Autodesk Inventor part; units mm, degrees
ref_plane "YZ Plane" through (0, 0, 0) normal (1, 0, 0) x (0, 1, 0)
ref_plane "XZ Plane" through (0, 0, 0) normal (0, 1, 0) x (-1, 0, 0)
ref_plane "XY Plane" through (0, 0, 0) normal (0, 0, 1) x (1, 0, 0)
sketch "Sketch1" plane through (0, 0, 0) normal (0, 1, 0) x (-1, 0, 0)
  line L0 (0, 0) -> (85.48, 0)
  line L1 (85.48, 0) -> (85.48, -127.76)
  line L2 (85.48, -127.76) -> (0, -127.76)
  line L3 (0, -127.76) -> (0, 0)
  line L4 (0, 0) -> (7.0711, -7.0711)
  line L5 (0, 0) -> (10, 0) construction
  circle A0 centre (7.0711, -7.0711) radius 4.7625
  dimension "d0" = 85.48
  dimension "d1" = 127.76
  dimension "offsetDiag" = 10
  dimension "d3" = 45
  dimension "d4" = 9.525
extrude "Extrusion1" add sketch "Sketch1" along normal blind 6.35 contours L0 L1 L2 L3 | A0
sketch "Sketch3" plane through (0, 6.35, 0) normal (0, 1, 0) x (1, 0, 0)
  line L0 (0, 0) -> (0, 127.76)
  line L1 (0, 0) -> (-2.3876, 0)
  line L2 (-2.3876, 0) -> (-2.3876, 9.8298)
  line L3 (-2.3876, 9.8298) -> (0, 9.8298)
  line L4 (0, 9.8298) -> (0, 0)
  line L5 (-2.3876, 9.8298) -> (-28.2876, 9.8298)
  line L6 (-28.2876, 9.8298) -> (-28.2876, 35.7298)
  line L7 (-28.2876, 35.7298) -> (-2.3876, 35.7298)
  line L8 (-2.3876, 35.7298) -> (-2.3876, 9.8298)
  line L9 (-28.2876, 35.7298) -> (-29.2876, 35.7298)
  line L10 (-29.2876, 35.7298) -> (-29.2876, 36.7298)
  line L11 (-29.2876, 36.7298) -> (-28.2876, 36.7298)
  line L12 (-28.2876, 36.7298) -> (-28.2876, 35.7298)
  dimension "d23" = 2.3876
  dimension "d24" = 9.8298
  dimension "d25" = 25.9
  dimension "d26" = 25.9
  dimension "d27" = 1
  dimension "d28" = 1
extrude "Extrusion2" cut sketch "Sketch3" against normal blind 1 contours L5 L6 L7 L8
pattern_linear "Rectangular Pattern2" count 3 spacing 27.4 along (-1, 0, 0) count 4 spacing 27.4 along (0, 0, -1) of "Extrusion2"
properties part number "inch substrate rack"
The listing builds one solid part. Answer for the finished solid, in the listing's coordinates (mm). A direction names the side the tool comes from. Give positions to 0.01 mm unless a question says otherwise; leave off trailing zeros. Order: outer loops, then holes, each group sorted by start corner. A loop starts at its lowest first (then second) coordinate and runs counter-clockwise, first axis right, second up.
Item 1: Find the intervals of material crossed by probe 1 along Z at (x, y) = (-26.5, 6); probe 2 along Y at (x, z) = (-10.5, -114), in increasing order.
From the geometry:
probe 1: z = -127.76 to -117.93, -92.03 to -90.53, -64.63 to -63.13, -37.23 to -35.73, -9.83 to 0
probe 2: y = 0 to 5.35
Item 2: Which of the six approach directions +Z, -Z, +X, -X, +Y, -Y give full straight-line access (tool end or side, diameter ignored) to faces 1 (the face through (-43, 5.35, -78)), 2 (the face through (-43, 3, -127.76))?
From the geometry:
face 1: +Y
face 2: -Z, +X, -X, +Y, -Y
Item 3: Given pin 1 Ø8 at (x, z) = (-39.5, -44.5) entering from +Y, flat-ended and moving along its own axis, determine where the tip first touches the part or whether it passes through.
From the geometry:
pin 1: stops at y = 5.35
Item 4: The part is cut by section A-A, the plane x = -8. Give the vertices of the cut face in (y, z), and give its area (3 significant figures).
From the geometry:
outline: (0, -127.76) - (6.35, -127.76) - (6.35, -117.93) - (5.35, -117.93) - (5.35, -92.03) - (6.35, -92.03) - (6.35, -90.53) - (5.35, -90.53) - (5.35, -64.63) - (6.35, -64.63) - (6.35, -63.13) - (5.35, -63.13) - (5.35, -37.23) - (6.35, -37.23) - (6.35, -35.73) - (5.35, -35.73) - (5.35, -9.83) - (6.35, -9.83) - (6.35, 0) - (0, 0) - close
area: 708 mm2
Item 5: The part is cut by section B-B, the plane z = -24.5. Give the vertices of the cut face in (x, y), and give its area (3 significant figures).
From the geometry:
outline: (-85.48, 0) - (0, 0) - (0, 6.35) - (-2.39, 6.35) - (-2.39, 5.35) - (-28.29, 5.35) - (-28.29, 6.35) - (-29.79, 6.35) - (-29.79, 5.35) - (-55.69, 5.35) - (-55.69, 6.35) - (-57.19, 6.35) - (-57.19, 5.35) - (-83.09, 5.35) - (-83.09, 6.35) - (-85.48, 6.35) - close
area: 465 mm2
